Can you work these out from the model? Positions are in its coordinate system, mm. A direction names the side the tool comes from. Coordinates: 2 decimals unless noted, no trailing zeros. Write each loop counter-clockwise with the first axis right and the second up, starting at its lowest first coordinate (ties: lowest second). Pieces come first, ordered by that corner, then holes. Notation, with made-up numbers: (25.25, -23) - (30.25, -23) arc R23 ccw to (30.25, 0) - close; hole circle Ø7 at (-19, 44). An arc over 180 degrees is marked (long way). Write each question's results on one line, items separated by ' | '. Start each with the question number.
```python
from build123d import *

# Parameters (mm, degrees)
EXTRUDE_1_DEPTH = 15
EXTRUDE_3_DEPTH = 89


with BuildPart() as part:
    # 草图1 → 凸台-拉伸1 (new body)
    with BuildSketch(Plane.XZ):
        Polygon((245, -50), (245, 50), (-245, 50), (-245, 35), (-235, 35), (-235, -35), (-245, -35), (-245, -50), align=None)
    extrude(amount=-EXTRUDE_1_DEPTH)

    # 草图2 → 凸台-拉伸3 (add)
    with BuildSketch(Plane.ZY.offset(235)):
        Polygon((-26.300861676, 7), (-35, 7), (-35, 15), (35, 15), (35, 7), align=None)
    extrude(amount=EXTRUDE_3_DEPTH)


solid = part.part
```
Q1. If we section it at A-A (y = 4): Please give me the cut outline in (x, z).
Q2. For faces 1 (the face through (-245, 7, 43)), 2 (the face through (-245, 7, -42)), 3 (the face through (-3, 7, -50)), which set-ups out of +Z, -Z, +X, -X, +Y, -Y let a thin tool reach every point of the face, with its end or its side?
Q3. I'm going to push flat-ended pins straight in: pin 1 Ø5 at (x, z) = (-267, -39.5) entering from -Y; pin 2 Ø6.5 at (x, y) = (-289.5, 12) entering from +Z; pin 3 Ø6.5 at (x, y) = (-287, 10.5) entering from -Z; pin 4 Ø2 at (y, z) = (4.5, -2) entering from -X. Where does each tip first touch, or does it pass through?
Q4. I need wall thicknesses on line 1 along X through (y, z) = (3.75, 37); line 2 along X through (y, z) = (4.5, -25); line 3 along Z through (x, y) = (-286, 9.75). Which ranges of each line are inside material? Lowest first, please. Write a range as from..to.
Q5. If we section it at B-B (z = 18): Please give me the cut outline in (x, y), then the cut area to 3 significant figures.
Answer list:
1) outline: (-245, -50) - (245, -50) - (245, 50) - (-245, 50) - (-245, 35) - (-235, 35) - (-235, -35) - (-245, -35) - close
2) face 1: +Z, -X, +Y, -Y | face 2: -Z, -X, +Y, -Y | face 3: -Z, +X, -X, +Y, -Y
3) pin 1: passes through | pin 2: stops at z = 35 | pin 3: stops at z = -35 | pin 4: stops at x = -235
4) line 1: x = -245..245 | line 2: x = -235..245 | line 3: z = -35..35
5) outline: (-324, 7) - (-235, 7) - (-235, 0) - (245, 0) - (245, 15) - (-324, 15) - close | area: 7,910 mm2
